The listing builds one solid part. Answer for the finished solid, in the listing's coordinates (mm). A direction names the side the tool comes from. Coordinates: 2 decimals unless noted, no trailing zeros. Write each loop counter-clockwise with the first axis right and the second up, starting at its lowest first coordinate (ties: lowest second). Pieces come first, ordered by that corner, then holes.
(1) The part is cut by section D-D on y = 45.5. Determine the outline of the cut face in (x, z).
(2) Given P1, Ø12, axis at x = -114, z = -28.5, coming from the -Y side; P2, Ø9, axis at y = 11.5, z = -16.5, coming from the -X side; P3, Ø2, axis at y = 53.5, z = -75.5, coming from the +X side, each flat-ended and moving along its own axis, determine where each tip first touches the part or whether it passes through.
(3) Which of the six approach directions +Z, -Z, +X, -X, +Y, -Y give full straight-line access (tool end or side, diameter ignored) to faces 5 (the flat face through (-172.668, 48, -8)), 6 (the flat face through (-3, 18, 140)), 7 (the flat face through (-2, 48, -123.522)), 8 (the flat face through (-3, 0, 129)), 9 (the flat face through (186.5, 18, 2))?
(4) For a pull along Z with two mould halves and no side action, classify faces 1 (the flat face through (-2, 48, 103.548)), 2 (the flat face through (-2, 2, 2)), 3 (the flat face through (-3, 18, -140)), 4 (the flat face through (-186.5, 18, 2)) as +Z half, -Z half, draft (parallel to the pull), parting line (faces both ways), or undercut.
(5) The part is cut by section C-C on y = 21.5. Determine the outline of the cut face in (x, z).
(6) The part is cut by section B-B on x = 119.5. Determine the outline of the cut face in (y, z).
(7) The part is cut by section A-A on z = 8. Determine the outline of the cut face in (x, y).
(8) Straight lines are drawn through the part: line 1 (Y direction, x = 146.5, z = -99); line 2 (X direction, y = 28, z = 126); line 3 (X direction, y = 55, z = -98.5). For each, find the intervals that lie inside material, in ascending order.
from build123d import *

# Parameters (mm, degrees)
SKETCH_1_W          = 390
SKETCH_1_H          = 295
EXTRUDE_1_DEPTH     = 3
SKETCH_2_W          = 373
SKETCH_2_H          = 280
EXTRUDE_2_DEPTH     = 30
SKETCH_4_W          = 345.33527023
SKETCH_4_H          = 227.069766727
EXTRUDE_3_DEPTH     = 30
SKETCH_5_W          = 304
SKETCH_5_H          = 229
CUT_EXTRUDE_4_DEPTH = 2


with BuildPart() as part:
    # 草图1 → 拉伸1 (new body)
    with BuildSketch(Plane(origin=(0, 0, 0), x_dir=(1, 0, 0), z_dir=(0, 1, 0))):
        Rectangle(SKETCH_1_W, SKETCH_1_H)
    extrude(amount=EXTRUDE_1_DEPTH)

    # 草图2 → 拉伸2 (add)
    with BuildSketch(Plane(origin=(0, 3, 0), x_dir=(1, 0, 0), z_dir=(0, 1, 0))):
        Rectangle(SKETCH_2_W, SKETCH_2_H)
    extrude(amount=EXTRUDE_2_DEPTH)

    # 草图4 → 拉伸3 (add)
    with BuildSketch(Plane(origin=(0, 33, 0), x_dir=(1, 0, 0), z_dir=(0, 1, 0))):
        with Locations((0, 9.986864741)):
            Rectangle(SKETCH_4_W, SKETCH_4_H)
    extrude(amount=EXTRUDE_3_DEPTH)

    # 草图5 → 拉伸4 (cut)
    with BuildSketch(Plane.XZ):
        Rectangle(SKETCH_5_W, SKETCH_5_H)
    extrude(amount=-CUT_EXTRUDE_4_DEPTH, mode=Mode.SUBTRACT)


solid = part.part
Model answer:
1. outline: (-172.67, -123.52) - (172.67, -123.52) - (172.67, 103.55) - (-172.67, 103.55) - close
2. P1: stops at y = 2
2. P2: stops at x = -186.5
2. P3: stops at x = 172.67
3. face 5: +Z, -Z, -X, +Y
3. face 6: +Z, +X, -X, +Y
3. face 7: -Z, +X, -X, +Y
3. face 8: +Z, -Z, +X, -X, -Y
3. face 9: +Z, -Z, +X, +Y
4. face 1: +Z half
4. face 2: undercut
4. face 3: -Z half
4. face 4: draft
5. outline: (-186.5, -140) - (186.5, -140) - (186.5, 140) - (-186.5, 140) - close
6. outline: (0, -147.5) - (3, -147.5) - (3, -140) - (33, -140) - (33, -123.52) - (63, -123.52) - (63, 103.55) - (33, 103.55) - (33, 140) - (3, 140) - (3, 147.5) - (0, 147.5) - (0, 114.5) - (2, 114.5) - (2, -114.5) - (0, -114.5) - close
7. outline: (-195, 0) - (-152, 0) - (-152, 2) - (152, 2) - (152, 0) - (195, 0) - (195, 3) - (186.5, 3) - (186.5, 33) - (172.67, 33) - (172.67, 63) - (-172.67, 63) - (-172.67, 33) - (-186.5, 33) - (-186.5, 3) - (-195, 3) - close
8. line 1: y = 2 to 63
8. line 2: x = -186.5 to 186.5
8. line 3: x = -172.67 to 172.67
